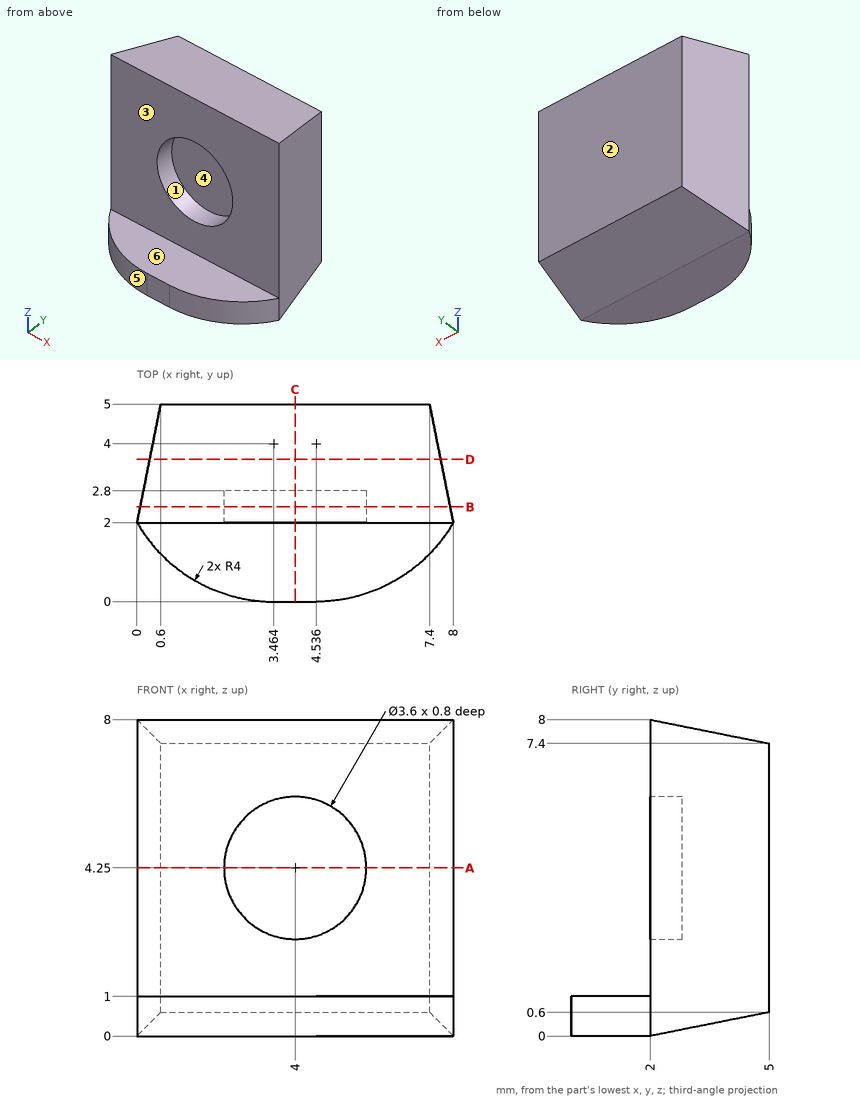
Answer from the drawing. Dimensions are ordinates in mm from the lowest x, y and z of the part. A direction names the side the tool comes from. Give positions to 0.01 mm unless a question says otherwise; leave off trailing zeros. Order: outer loops, then holes, each group sorted by start corner. A loop starts at its lowest first (then second) coordinate and runs counter-clockwise, first axis right, second up. Notation, with made-up numbers: (20.25, -6) -> (79.25, -6) arc R29 ccw to (79.25, 27) -> close; hole circle Ø10 at (79, -16.75). An arc over 180 degrees is marked (long way). One line per item, written item: value. Start each with the question number.
(1) Flat-ended cylindrical pins translate along their axes: P1, Ø2, axis at x = 5, z = 2.5, coming from the -Y side; P2, Ø1, axis at x = 3.5, y = 3, coming from the -Z side; P3, Ø2, axis at y = 3.5, z = 2.5, coming from the -X side. Find the tip coordinate at first contact, or state that the pin passes through.
(2) A tool of negligible diameter and unlimited length cuts with its end or side. For the marked faces 1, 2 and 3, from which of +Z, -Z, +X, -X, +Y, -Y can it reach the whole face along a straight path? Write none if from no direction.
(3) The part is cut by section C-C (x = 4). Determine the outline of the cut face in (y, z).
(4) For a pull along X with two mould halves and no side action, classify the marked faces 4, 5 and 6 as released by +X, released by -X, zero draft, split by the parting line, or undercut.
(5) Straight lines are drawn through the part: L1, parallel to Y at x = 5.5, z = 1.5; L2, parallel to X at y = 2.4, z = 4.25; L3, parallel to Y at x = 3.75, z = 3.5. For each, find the intervals that lie inside material, in ascending order.
(6) The part is cut by section B-B (y = 2.4). Determine the outline of the cut face in (x, z).
(7) The part is cut by section A-A (z = 4.25). Determine the outline of the cut face in (x, y).
(8) The part is cut by section D-D (y = 3.6). Determine the outline of the cut face in (x, z), and give its area (3 significant figures).
Taken from the geometry:
1. P1: y = 2
1. P2: z = 0.1
1. P3: x = 0.1
2. face 1: -Y
2. face 2: +Z, -Z, +X, -X, +Y
2. face 3: +Z, +X, -X, -Y
3. outline: (0, 0) -> (2, 0) -> (5, 0.6) -> (5, 7.4) -> (2, 8) -> (2, 6.05) -> (2.8, 6.05) -> (2.8, 2.45) -> (2, 2.45) -> (2, 1) -> (0, 1) -> close
4. face 4: undercut
4. face 5: released by -X
4. face 6: zero draft
5. L1: 2 to 5
5. L2: 0.08 to 2.2, 5.8 to 7.92
5. L3: 2.8 to 5
6. outline: (0.08, 0.08) -> (7.92, 0.08) -> (7.92, 7.92) -> (0.08, 7.92) -> close; hole circle Ø3.6 at (4, 4.25)
7. outline: (0, 2) -> (2.2, 2) -> (2.2, 2.8) -> (5.8, 2.8) -> (5.8, 2) -> (8, 2) -> (7.4, 5) -> (0.6, 5) -> close
8. outline: (0.32, 0.32) -> (7.68, 0.32) -> (7.68, 7.68) -> (0.32, 7.68) -> close
8. area: 54.2 mm^2
